Could you check a few things on this model? Use its own coordinates, in mm. A direction names the side the tool comes from. Coordinates: 2 decimals unless noted, no trailing zeros. Write each loop counter-clockwise with the first axis right and the second up, starting at its lowest first coordinate (ties: lowest second). Pieces come first, ordered by that corner, then holes.
```python
from build123d import *

# Parameters (mm, degrees)
F0_W      = 101.6
F0_H      = 50.8
F1_DEPTH  = 0.2
F2_W      = 88.9
F2_H      = 50.8
F3_DEPTH  = 0.2
F4_W      = 76.2
F4_H      = 50.8
F5_DEPTH  = 0.4
F6_W      = 63.5
F6_H      = 50.8
F7_DEPTH  = 0.8
F8_W      = 50.8
F8_H      = 50.8
F9_DEPTH  = 0.8
F10_W     = 0.4
F10_H     = 50.8
F10_W_2   = 0.8
F10_W_3   = 1.2
F10_W_4   = 1.6
F11_DEPTH = 12.7


with BuildPart() as f1:
    # F0 (on Top) → F1 (new body)
    with BuildSketch(Plane.XY):
        Rectangle(F0_W, F0_H)
    extrude(amount=F1_DEPTH)

    # F2 (on face) → F3 (join)
    with BuildSketch(Plane.XY.offset(0.2)):
        with Locations((6.35, 0)):
            Rectangle(F2_W, F2_H)
    extrude(amount=F3_DEPTH)

    # F4 (on face) → F5 (join)
    with BuildSketch(Plane.XY.offset(0.4)):
        with Locations((12.7, 0)):
            Rectangle(F4_W, F4_H)
    extrude(amount=F5_DEPTH)

    # F6 (on face) → F7 (join)
    with BuildSketch(Plane.XY.offset(0.8)):
        with Locations((19.05, 0)):
            Rectangle(F6_W, F6_H)
    extrude(amount=F7_DEPTH)

    # F8 (on face) → F9 (join)
    with BuildSketch(Plane.XY.offset(1.6)):
        with Locations((25.4, 0)):
            Rectangle(F8_W, F8_H)
    extrude(amount=F9_DEPTH)

    # F10 (on face) → F11 (join)
    with BuildSketch(Plane.XY.offset(2.4)):
        with Locations((12.9, 0)):
            Rectangle(F10_W, F10_H)
        with Locations((26.2, 0)):
            Rectangle(F10_W_2, F10_H)
        with Locations((39.9, 0)):
            Rectangle(F10_W_3, F10_H)
        with Locations((50, 0)):
            Rectangle(F10_W_4, F10_H)
    extrude(amount=F11_DEPTH)


solid = f1.part
```
1. I want a section at B-B on y = 18. Please give me the cut outline in (x, z).
Verdict:
outline: (-50.8, 0) - (50.8, 0) - (50.8, 15.1) - (49.2, 15.1) - (49.2, 2.4) - (40.5, 2.4) - (40.5, 15.1) - (39.3, 15.1) - (39.3, 2.4) - (26.6, 2.4) - (26.6, 15.1) - (25.8, 15.1) - (25.8, 2.4) - (13.1, 2.4) - (13.1, 15.1) - (12.7, 15.1) - (12.7, 2.4) - (0, 2.4) - (0, 1.6) - (-12.7, 1.6) - (-12.7, 0.8) - (-25.4, 0.8) - (-25.4, 0.4) - (-38.1, 0.4) - (-38.1, 0.2) - (-50.8, 0.2) - close
2. For pin 1 (12 mm diameter, centred on x = 35, y = 5, fed in from -Z); pin 2 (1.5 mm diameter, centred on x = 22, y = 11, fed in from +Z); pin 3 (6.5 mm diameter, centred on x = -45, y = -9, fed in from +Z); pin 4 (6.5 mm diameter, centred on x = -20, y = -1, fed in from +Z), each with a flat end and sliding along its axis, tell me the tip position at first contact or that it passes through.
Verdict:
pin 1: stops at z = 0
pin 2: stops at z = 2.4
pin 3: stops at z = 0.2
pin 4: stops at z = 0.8
3. I want a section at C-C on x = -29.5. Please give me the cut outline in (y, z).
Verdict:
outline: (-25.4, 0) - (25.4, 0) - (25.4, 0.4) - (-25.4, 0.4) - close
4. I want a section at A-A on z = 5.25. Please give me the cut outline in (x, y), plus the area to 3 significant figures.
Verdict:
outline: (12.7, -25.4) - (13.1, -25.4) - (13.1, 25.4) - (12.7, 25.4) - close; (25.8, -25.4) - (26.6, -25.4) - (26.6, 25.4) - (25.8, 25.4) - close; (39.3, -25.4) - (40.5, -25.4) - (40.5, 25.4) - (39.3, 25.4) - close; (49.2, -25.4) - (50.8, -25.4) - (50.8, 25.4) - (49.2, 25.4) - close
area: 203 mm2
5. Please list where these lines run through material, in increasing order: line 1 along X through (y, z) = (-14, 4); line 2 along Z through (x, y) = (-32.5, 20.5); line 3 along Z through (x, y) = (-22, 3).
Verdict:
line 1: x = 12.7 to 13.1, 25.8 to 26.6, 39.3 to 40.5, 49.2 to 50.8
line 2: z = 0 to 0.4
line 3: z = 0 to 0.8
6. If we mould it in two halves opening along X, with no side actions, what happens to faces 1 (the face through (39.3, 0, 9)), 2 (the face through (50.8, 0, 7)), 3 (the face through (-6, 0, 1.6))? For each: pulls with the +X half, pulls with the -X half, needs draft (parallel to the pull), parting line crosses it, or undercut.
Verdict:
face 1: undercut
face 2: pulls with the +X half
face 3: needs draft
7. On a 3-axis mill with a long thin cutter (end or side, diameter ignored), from which of +Z, -Z, +X, -X, +Y, -Y can I reach the whole of each face in a straight line? I mean faces 4 (the face through (-32, 0, 0.4)), 5 (the face through (-1, 0, 0)), 6 (the face through (13.1, 0, 9)). Say none if no direction works.
Verdict:
face 4: +Z, -X, +Y, -Y
face 5: -Z, +X, -X, +Y, -Y
face 6: +Z, +Y, -Y
8. I want a section at D-D on x = 16. Please give me the cut outline in (y, z), plus the area to 3 significant figures.
Verdict:
outline: (-25.4, 0) - (25.4, 0) - (25.4, 2.4) - (-25.4, 2.4) - close
area: 122 mm2
